Verification items for the finished model (mm, model axes). Face numbers are marked on the shaded views. A direction names the side the tool comes from. Coordinates: 2 decimals unless noted, no trailing zeros. Order: outer loops, then holes, each group sorted by start corner. A loop starts at its lowest first (then second) coordinate and runs counter-clockwise, first axis right, second up. Notation, with made-up numbers: M -33.75,-8.5 L -9.75,-8.5 A12 ccw -9.75,0.5 Z; hole C 66,-5.5 d4. An arc over 180 degrees is marked long. Return JSON: item names as keys, results as strings.
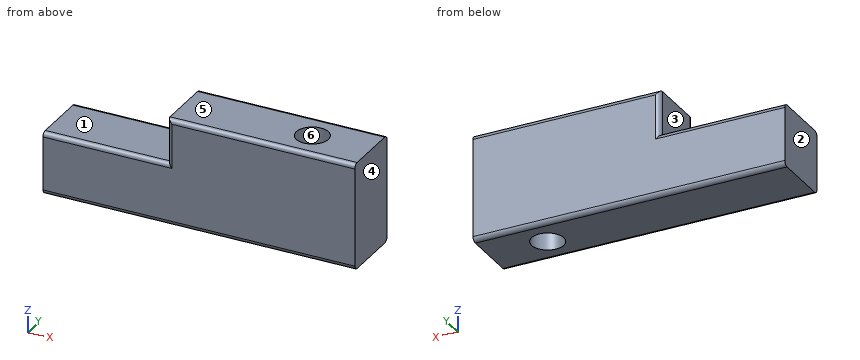
```python
from build123d import *

# Parameters (mm, degrees)
SKETCH1_W                  = 35
SKETCH1_H                  = 7
BOSS_EXTRUDE1_DEPTH        = 7
SKETCH3_W                  = 21
SKETCH3_H                  = 7
BOSS_EXTRUDE3_DEPTH        = 5
FILLET1_R                  = 0.5
F_3_6_3_6_DIAMETER_HOLE1_D = 3.6


with BuildPart() as part:
    # Sketch1 → Boss-Extrude1 (new body)
    with BuildSketch(Plane.XY):
        Rectangle(SKETCH1_W, SKETCH1_H)
    extrude(amount=BOSS_EXTRUDE1_DEPTH)

    # Sketch3 → Boss-Extrude3 (add)
    with BuildSketch(Plane.XY.offset(7)):
        with Locations((7, 0)):
            Rectangle(SKETCH3_W, SKETCH3_H)
    extrude(amount=BOSS_EXTRUDE3_DEPTH)

    # Fillet1
    fillet1_edges = [part.edges().sort_by_distance(p)[0] for p in [
        (-10.5, 3.5, 7),
        (-3.5, 3.5, 9.5),
        (-3.5, -3.5, 9.5),
        (-10.5, -3.5, 7),
        (7, 3.5, 12),
        (7, -3.5, 12),
        (0, -3.5, 0),
        (0, 3.5, 0),
    ]]
    fillet(fillet1_edges, radius=FILLET1_R)

    # Ø3.6 (3.6) Diameter Hole1 (through all)
    with Locations(Plane(origin=(10.929593105, 0, 0), x_dir=(-1, 0, 0), z_dir=(0, 0, -1))):
        with Locations((0, 0)):
            Hole(F_3_6_3_6_DIAMETER_HOLE1_D / 2)


solid = part.part
```
Q1. Cross-section at C-C, the plane x = -11. Record the boundary of the cut face in (y, z).
Values:
{"outline": "M -3.5,0.5 A0.5 ccw -3,0 L 3,0 A0.5 ccw 3.5,0.5 L 3.5,6.5 A0.5 ccw 3,7 L -3,7 A0.5 ccw -3.5,6.5 Z"}
Q2. Material ranges on line 1 along Y through (x, z) = (11, 7.75); line 2 along X through (y, z) = (-3, 9); line 3 along Z through (x, y) = (-12.5, 1), recorded low to high.
Values:
{"line 1": "-3.5 to -1.8, 1.8 to 3.5", "line 2": "-3.5 to 17.5", "line 3": "0 to 7"}
Q3. Cross-section at A-A, the plane y = 0. Record the boundary of the cut face in (x, z), and give its area (3 significant figures).
Values:
{"outline": "M -17.5,0 L 9.13,0 L 9.13,12 L -3.5,12 L -3.5,7 L -17.5,7 Z; M 12.73,0 L 17.5,0 L 17.5,12 L 12.73,12 Z", "area": "307 mm^2"}
Q4. Tool access check on the marked faces 1 and 2. Record the directions out of +Z, -Z, +X, -X, +Y, -Y that give a thin tool (end or side, any length) a straight path to the whole face; none if there is none.
Values:
{"face 1": "+Z, -X, +Y, -Y", "face 2": "+Z, -Z, -X, +Y, -Y"}
Q5. Cross-section at D-D, the plane y = -2.5. Record the boundary of the cut face in (x, z).
Values:
{"outline": "M -17.5,0 L 17.5,0 L 17.5,12 L -3.5,12 L -3.5,7 L -17.5,7 Z"}
Q6. Go/stop test with flat-tipped pins: pin 1 (2.5 mm diameter, centred on y = 0, z = 10.5, fed in from -X); pin 2 (3 mm diameter, centred on x = -5.5, y = -1, fed in from +Z). Record where each tip stops, or that it passes through.
Values:
{"pin 1": "x = -3.5", "pin 2": "z = 7"}
Q7. Draft check along X on the marked faces 3, 4, 5 and 6. Enter one of: pulls with the +X half, pulls with the -X half, needs draft (parallel to the pull), parting line crosses it, or undercut.
Values:
{"face 3": "pulls with the -X half", "face 4": "pulls with the +X half", "face 5": "needs draft", "face 6": "undercut"}
Q8. Cross-section at B-B, the plane z = 8. Record the boundary of the cut face in (x, y).
Values:
{"outline": "M -3.5,-3 A0.5 ccw -3,-3.5 L 17.5,-3.5 L 17.5,3.5 L -3,3.5 A0.5 ccw -3.5,3 Z; hole C 10.93,0 d3.6"}
